```python
from build123d import *

# Parameters (mm, degrees)
SKETCH1_W           = 23
SKETCH1_H           = 40
BOSS_EXTRUDE1_DEPTH = 3
SKETCH2_R           = 4.1
CUT_EXTRUDE1_DEPTH  = 3
SKETCH3_W           = 12
SKETCH3_H           = 3
BOSS_EXTRUDE2_DEPTH = 40
SKETCH4_W           = 2.5
SKETCH4_H           = 12
BOSS_EXTRUDE3_DEPTH = 6
SKETCH6_W           = 8
SKETCH6_H           = 10
BOSS_EXTRUDE4_DEPTH = 2.5
SKETCH7_R           = 2
CUT_EXTRUDE2_DEPTH  = 78.511007161


with BuildPart() as part:
    # Sketch1 → Boss-Extrude1 (new body)
    with BuildSketch(Plane.XY):
        with Locations((0, 20)):
            Rectangle(SKETCH1_W, SKETCH1_H)
    extrude(amount=-BOSS_EXTRUDE1_DEPTH)

    # Sketch2 → Cut-Extrude1 (cut)
    with BuildSketch(Plane.XY):
        with Locations((0, 34)):
            Circle(SKETCH2_R)
    extrude(amount=-CUT_EXTRUDE1_DEPTH, mode=Mode.SUBTRACT)

    # Sketch3 → Boss-Extrude2 (add)
    with BuildSketch(Plane(origin=(0, 40, 0), x_dir=(1, 0, 0), z_dir=(0, 1, 0))):
        with Locations((0, 1.5)):
            Rectangle(SKETCH3_W, SKETCH3_H)
    extrude(amount=BOSS_EXTRUDE2_DEPTH)

    # Sketch4 → Boss-Extrude3 (add)
    with BuildSketch(Plane(origin=(0, 0, -3), x_dir=(-1, 0, 0), z_dir=(0, 0, -1))):
        with Locations((-10.25, 6)):
            Rectangle(SKETCH4_W, SKETCH4_H)
    extrude(amount=BOSS_EXTRUDE3_DEPTH)

    # Sketch6 → Boss-Extrude4 (add)
    with BuildSketch(Plane(origin=(24.104535363, 66.226666617, 0), x_dir=(0, 0, -1), z_dir=(0.34202014332566943, 0.9396926207859081, 0))):
        with Locations((7, 36.228956157)):
            Rectangle(SKETCH6_W, SKETCH6_H)
    extrude(amount=BOSS_EXTRUDE4_DEPTH)

    # Sketch7 → Cut-Extrude2 (cut, through all)
    with BuildSketch(Plane(origin=(24.104535363, 66.226666617, 0), x_dir=(0.9396926207859078, -0.3420201433256706, 0), z_dir=(-0.3420201433256706, -0.9396926207859078, 0))):
        with Locations((-36.228956157, -8)):
            Circle(SKETCH7_R)
    extrude(amount=-CUT_EXTRUDE2_DEPTH, mode=Mode.SUBTRACT)


solid = part.part
```
Read the model definition and answer for the solid it produces. Units are mm, in the model's axes. A direction names the side the tool comes from. Coordinates: 2 decimals unless noted, no trailing zeros. Loops run counter-clockwise (first coordinate to the right, second up) from the corner with the lowest first, then second, coordinate; pieces in that order, holes last.
(1) The mould has two halves that part along X. Classify faces 1 (the face through (-10, 80, -3)), 2 (the face through (-6, 60, -1)), 3 (the face through (-3.022, 36.771, -1.479)): released by +X, released by -X, zero draft, split by the parting line, or undercut.
Solution:
face 1: zero draft
face 2: released by -X
face 3: undercut
(2) Flat-ended cylindrical pins translate along their axes: pin 1 Ø10 at (x, y) = (7, 36) entering from -Z; pin 2 Ø0.9 at (x, z) = (9, -2) entering from +Y; pin 3 Ø5 at (x, y) = (-7, 11.5) entering from +Z; pin 4 Ø0.9 at (y, z) = (23, -1) entering from -X. Find the tip coordinate at first contact, or state that the pin passes through.
Solution:
pin 1: stops at z = -3
pin 2: stops at y = 40
pin 3: stops at z = 0
pin 4: stops at x = -11.5
(3) The part is cut by section D-D (y = 14). Determine the outline of the cut face in (x, z).
Solution:
outline: (-11.5, -3) - (11.5, -3) - (11.5, 0) - (-11.5, 0) - close
(4) Consider line 1 along Y through (x, z) = (0, -0.95); line 2 along Z through (x, y) = (3.75, 68); line 3 along X through (y, z) = (51.5, -2.25). Determine where each line is inside the solid, lowest interval first.
Solution:
line 1: y = 0 to 29.9, 38.1 to 80
line 2: z = -3 to 0
line 3: x = -6 to 6
(5) The part is cut by section C-C (z = -6.75). Determine the outline of the cut face in (x, y).
Solution:
outline: (-14.64, 80.33) - (-11.41, 79.15) - (-10.55, 81.5) - (-13.78, 82.68) - close; (-8.47, 78.08) - (-5.24, 76.91) - (-4.39, 79.26) - (-7.62, 80.43) - close; (9, 0) - (11.5, 0) - (11.5, 12) - (9, 12) - close
(6) A tool of negligible diameter and unlimited length cuts with its end or side. For faces 4 (the face through (-10.19, 81.37, -6.06)), 5 (the face through (-4.82, 78.07, -6.94)), 6 (the face through (-9, 40, -1)), from which of +Z, -Z, +X, -X, +Y, -Y can it reach the whole face along a straight path? Write none if from no direction.
Solution:
face 4: -Z, +X, +Y
face 5: -Z, +X, -Y
face 6: +Z, -Z, -X, +Y
(7) The part is cut by section A-A (y = 34). Determine the outline of the cut face in (x, z), and give its area (3 significant figures).
Solution:
outline: (-11.5, -3) - (-4.1, -3) - (-4.1, 0) - (-11.5, 0) - close; (4.1, -3) - (11.5, -3) - (11.5, 0) - (4.1, 0) - close
area: 44.4 mm2
(8) The part is cut by section B-B (x = 0). Determine the outline of the cut face in (y, z), and give its area (3 significant figures).
Solution:
outline: (0, -3) - (29.9, -3) - (29.9, 0) - (0, 0) - close; (38.1, -3) - (80, -3) - (80, 0) - (38.1, 0) - close
area: 215 mm2
